The listing builds one solid part. Answer for the finished solid, in the listing's coordinates (mm). A direction names the side the tool comes from. Coordinates: 2 decimals unless noted, no trailing zeros. Loops run counter-clockwise (first coordinate to the right, second up) from the corner with the lowest first, then second, coordinate; pieces in that order, holes last. Notation, with made-up numbers: (18.25, 26) - (66.25, 26) arc R19 cw to (66.25, 45) - close; hole circle Ø1 at (36, -21). An arc over 180 degrees is marked (long way). Put each result on its own line as item: value.
Autodesk Inventor part; units mm, degrees
ref_plane "YZ Plane" through (0, 0, 0) normal (1, 0, 0) x (0, 1, 0)
ref_plane "XZ Plane" through (0, 0, 0) normal (0, 1, 0) x (-1, 0, 0)
ref_plane "XY Plane" through (0, 0, 0) normal (0, 0, 1) x (1, 0, 0)
sketch "Sketch1" plane through (0, 0, 0) normal (0, 0, 1) x (1, 0, 0)
  line L0 (0, 0) -> (15, 0)
  line L1 (15, 0) -> (15, 20)
  line L2 (15, 20) -> (0, 20)
  line L3 (0, 20) -> (0, 0)
  line L4 (0, 3) -> (15, 3)
  line L5 (15, 3) -> (15, 17)
  line L6 (15, 17) -> (0, 17)
  line L7 (0, 17) -> (0, 3)
  line L8 (0, 3) -> (15, 17) construction
  line L9 (15, 3) -> (0, 17) construction
  arc A0 (15, 17) -> (0, 17) centre (7.5, 9.125) ccw
  arc A1 (0, 3) -> (15, 3) centre (7.5, 10.875) ccw
  line L10 (-1.5875, -1.5875) -> (16.5875, -1.5875)
  line L11 (16.5875, -1.5875) -> (16.5875, 21.5875)
  line L12 (16.5875, 21.5875) -> (-1.5875, 21.5875)
  line L13 (-1.5875, 21.5875) -> (-1.5875, -1.5875)
  arc A2 (18.2337, 15.4576) -> (-3.6211, 14.7494) centre (7.5, 9.125) ccw
  line L14 (7.5, 10) -> (5.1883, 10)
  arc A3 (-3.6211, 5.2506) -> (18.2337, 4.5424) centre (7.5, 10.875) ccw
  point P0 (16.5875, 2.3467)
  point P1 (16.5875, 17.6533)
  point P2 (-1.5875, 17.6533)
  point P3 (-1.5875, 2.3467)
  dimension "d2" = 15
  dimension "d3" = 20
  dimension "d4" = 14
  dimension "d5" = 7.5
  dimension "d6" = 10
  dimension "d7" = 1.5875
  dimension "d8" = 1.5875
extrude "Extrusion1" add sketch "Sketch1" along normal blind 6.35 contours A3 L3 A1 L0 | L0 A3 | A3 L13 A2 L3 | A1 L1 A3 L0 | L1 A2 L11 A3 | L3 A2 L2 A0 | A0 L2 A2 L1 | L2 A2
properties part number "motor_holder_test_fit"
1) Straight lines are drawn through the part: L1, parallel to X at y = 14.75, z = 4.5; L2, parallel to Y at x = 4.5, z = 2.25; L3, parallel to Y at x = 8.75, z = 1. For each, find the intervals that lie inside material, in ascending order. Write a range as [from, to].
Found:
L1: x = [-1.59, 0], [15, 16.59]
L2: y = [-1.22, 0.42], [19.58, 21.22]
L3: y = [-1.52, 0.07], [19.93, 21.52]
2) The part is cut by section C-C (x = 0.25). Give the vertices of the cut face in (y, z).
Found:
outline: (0.74, 0) - (2.77, 0) - (2.77, 6.35) - (0.74, 6.35) - close; (17.23, 0) - (19.26, 0) - (19.26, 6.35) - (17.23, 6.35) - close
3) For a pull along X with two mould halves and no side action, classify faces 3 (the face through (-1, 10, 0)), 4 (the face through (-1.588, 10, 3)), 5 (the face through (7.4, 20, 3.1)), 6 (the face through (15, 10, 3)) as pulls with the +X half, pulls with the -X half, needs draft (parallel to the pull), parting line crosses it, or undercut.
Found:
face 3: needs draft
face 4: pulls with the -X half
face 5: undercut
face 6: undercut
4) For faces 1 (the face through (7.357, 21.587, 3.131)), 2 (the face through (7.6, 0, 3.1)), determine the directions among +Z, -Z, +X, -X, +Y, -Y from which every point of the face is accessible in a straight line to the end or side of a thin tool.
Found:
face 1: +Z, -Z, +Y
face 2: +Z, -Z
5) Each of these flat-tipped pins is pushed along its axis until it touches: pin 1 (1 mm diameter, centred on x = 10, y = 1, fed in from -Z); pin 2 (1.5 mm diameter, centred on y = 18.5, z = 3, fed in from -X). Where does it stop, or does it pass through?
Found:
pin 1: passes through
pin 2: stops at x = -1.5
6) The part is cut by section A-A (y = 16). Give the vertices of the cut face in (x, z).
Found:
outline: (-1.59, 0) - (0, 0) - (0, 6.35) - (-1.59, 6.35) - close; (15, 0) - (16.59, 0) - (16.59, 6.35) - (15, 6.35) - close
